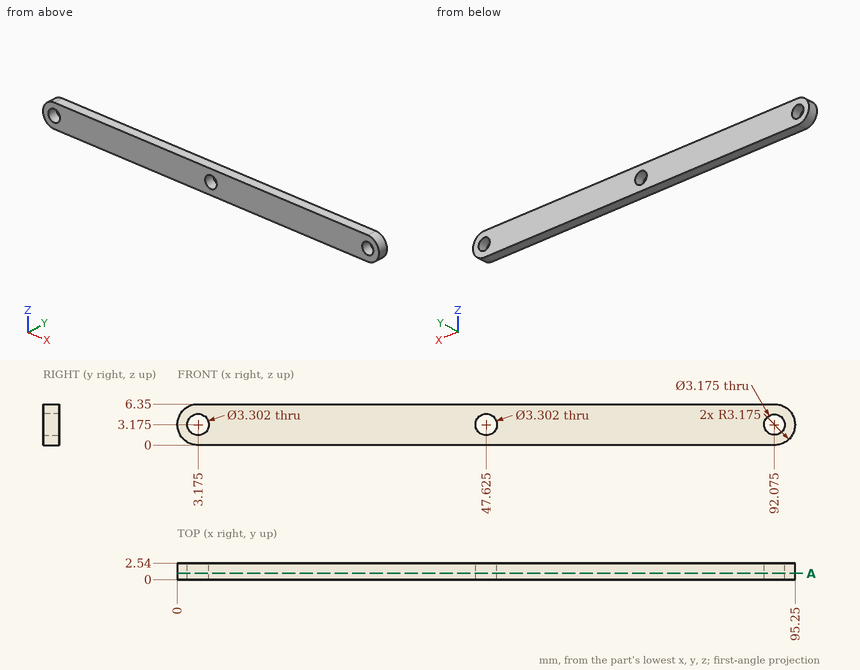
Print and shaded views of the part. All mm, measured from the part's lowest x, y and z. Give positions to 0.01 mm unless a question says otherwise; leave off trailing zeros. Put each result on its own line as item: value.
(1) Saw through at A-A (y = 0.95). Count the separate pieces of the cut face and the enclosed holes in it, then the cut area to 3 significant figures.
Working result:
separate pieces: 1
enclosed holes: 3
area: 571 mm^2
(2) Wall check: L1, parallel to X at y = 2.35, z = 3.5; L2, parallel to X at y = 2.05, z = 5; L3, parallel to X at y = 1.05, z = 0.5. Give the ranges that are in metal, low to high.
Working result:
L1: 0.02 to 1.56, 4.79 to 46.01, 49.24 to 90.52, 93.63 to 95.23
L2: 0.58 to 94.67
L3: 1.46 to 93.79
(3) Drop a flat-ended pin along its axis: pin 1 Ø1 at (y, z) = (1.5, 2.5) entering from +X. Give the stop position or say it passes through.
Working result:
pin 1: x = 95.25
